from build123d import *

# Parameters (mm, degrees)
BOSS_EXTRUDE1_DEPTH = 15.86
SKETCH3_R           = 2.35
BOSS_EXTRUDE2_DEPTH = 1.8
SKETCH4_R           = 2.35
BOSS_EXTRUDE3_DEPTH = 1.8
SHELL1_T            = -1.4
SKETCH5_R           = 2.45
SKETCH5_R_2         = 1.45
BOSS_EXTRUDE4_DEPTH = 1.8
SKETCH6_R           = 3.05
SKETCH6_R_2         = 2.395
BOSS_EXTRUDE5_DEPTH = 1.55


with BuildPart() as part:
    # Sketch2 → Boss-Extrude1 (new body)
    with BuildSketch(Plane(origin=(0, 0, 0), x_dir=(0, 0, -1), z_dir=(1, 0, 0))):
        Polygon((0, 0), (0, 6.35), (-7.81, 6.35), (-7.81, 3.15), (-15.86, 3.15), (-15.86, 0), align=None)
    extrude(amount=BOSS_EXTRUDE1_DEPTH)

    # Sketch3 → Boss-Extrude2 (add)
    with BuildSketch(Plane(origin=(0, 6.35, 0), x_dir=(1, 0, 0), z_dir=(0, 1, 0))):
        with Locations(Location((3.98, -3.98, 0), (0, 0, 90))):
            Circle(SKETCH3_R)
        with Locations(Location((11.88, -3.98, 0), (0, 0, 90))):
            Circle(SKETCH3_R)
    extrude(amount=BOSS_EXTRUDE2_DEPTH)

    # Sketch4 → Boss-Extrude3 (add)
    with BuildSketch(Plane(origin=(0, 3.15, 0), x_dir=(1, 0, 0), z_dir=(0, 1, 0))):
        with Locations(Location((3.98, -11.88, 0), (0, 0, 90))):
            Circle(SKETCH4_R)
        with Locations(Location((11.88, -11.88, 0), (0, 0, 90))):
            Circle(SKETCH4_R)
    extrude(amount=BOSS_EXTRUDE3_DEPTH)

    # Shell1
    shell1_openings = [part.faces().sort_by_distance(p)[0] for p in [
        (7.93, 0, 7.93),
    ]]
    offset(amount=SHELL1_T, openings=shell1_openings, kind=Kind.INTERSECTION)

    # Sketch5 → Boss-Extrude4 (add)
    # profile 1 of 2: a face of its own
    with BuildSketch(Plane(origin=(0, 0, 0), x_dir=(-1, 0, 0), z_dir=(0, 0, -1))):
        with Locations(Location((-11.88, 3.9, 0), (0, 0, 90))):
            Circle(SKETCH5_R)
        with Locations((-11.88, 3.9)):
            Circle(SKETCH5_R_2, mode=Mode.SUBTRACT)
    # profile 2 of 2: a face of its own
    with BuildSketch(Plane(origin=(0, 0, 0), x_dir=(-1, 0, 0), z_dir=(0, 0, -1))):
        with Locations(Location((-3.92, 3.9, 0), (0, 0, 90))):
            Circle(SKETCH5_R)
        with Locations((-3.92, 3.9)):
            Circle(SKETCH5_R_2, mode=Mode.SUBTRACT)
    extrude(amount=BOSS_EXTRUDE4_DEPTH)

    # Sketch6 → Boss-Extrude5 (add)
    with BuildSketch(Plane.XZ.offset(-1.75)):
        with Locations(Location((7.93, 7.93, 0), (0, 0, 90))):
            Circle(SKETCH6_R)
        with Locations(Location((7.93, 7.93, 0), (0, 0, 90))):
            Circle(SKETCH6_R_2, mode=Mode.SUBTRACT)
    extrude(amount=BOSS_EXTRUDE5_DEPTH)


solid = part.part
Work out the finished part from the listing and answer in its coordinate system (mm). A direction names the side the tool comes from. Give positions to 0.01 mm unless a question says otherwise; leave off trailing zeros. Order: outer loops, then holes, each group sorted by start corner. A loop starts at its lowest first (then second) coordinate and runs counter-clockwise, first axis right, second up. Notation, with made-up numbers: (-31, 88.25) -> (-3, 88.25) arc R10 cw to (-3, 95.25) -> close; hole circle Ø7 at (77.5, 66). An arc over 180 degrees is marked (long way). Answer as a JSON object with one key per item and string values. Group by question number.
1. Section B-B on x = 7.93 is taken. Determine the outline of the cut face in (y, z) (3 decimals), plus the area to 3 significant figures.
2. Section A-A on y = 3.9 is taken. Determine the outline of the cut face in (x, z), plus the area to 3 significant figures.
3. The mould has two halves that part along Z. Classify faces 1 (the flat face through (8, 2, 0)), 2 (the cylindrical face through (7.01, 0.99, 10.84)), 3 (the flat face through (8, 4.95, 4)), 4 (the cylindrical face through (1.53, 3.37, -0.89)): released by +Z, released by -Z, zero draft, split by the parting line, or undercut.
4. Flat-ended cylindrical pins translate along their axes: pin 1 Ø1.9 at (x, y) = (9, 0.5) entering from -Z; pin 2 Ø1.5 at (x, z) = (5, 4) entering from -Y; pin 3 Ø3 at (x, z) = (10, 8) entering from -Y. Find the tip coordinate at first contact, or state that the pin passes through.
5. Section C-C on z = -0.5 is taken. Determine the outline of the cut face in (x, y), plus the area to 3 significant figures.
6. A tool of negligible diameter and unlimited length cuts with its end or side. For faces 5 (the flat face through (4, 3.55, 12)), 6 (the cylindrical face through (13.965, 4.037, 10.796)), 7 (the flat face through (4, 4, 0)), from which of +Z, -Z, +X, -X, +Y, -Y can it reach the whole face along a straight path? Write none if from no direction.
7. Section D-D on z = 3.98 is taken. Determine the outline of the cut face in (x, y).
8. Consider line 1 along X through (y, z) = (5.7, 3.98); line 2 along Z through (x, y) = (4.5, 3); line 3 along X through (y, z) = (1.25, 12.25). Determine where each line is inside the solid, lowest interval first. Write a range as [from, to].
Result sheet:
{
 "1": {"outline": "(0, 0) -> (6.35, 0) -> (6.35, 7.81) -> (3.15, 7.81) -> (3.15, 15.86) -> (0, 15.86) -> (0, 14.46) -> (1.75, 14.46) -> (1.75, 10.98) -> (0.2, 10.98) -> (0.2, 10.325) -> (1.75, 10.325) -> (1.75, 6.41) -> (4.95, 6.41) -> (4.95, 1.4) -> (0, 1.4) -> close; (0.2, 4.88) -> (1.75, 4.88) -> (1.75, 5.535) -> (0.2, 5.535) -> close", "area": "38.1 mm^2"},
 "2": {"outline": "(0, 0) -> (1.47, 0) -> (1.47, -1.8) -> (2.47, -1.8) -> (2.47, 0) -> (5.37, 0) -> (5.37, -1.8) -> (6.37, -1.8) -> (6.37, 0) -> (9.43, 0) -> (9.43, -1.8) -> (10.43, -1.8) -> (10.43, 0) -> (13.33, 0) -> (13.33, -1.8) -> (14.33, -1.8) -> (14.33, 0) -> (15.86, 0) -> (15.86, 7.81) -> (0, 7.81) -> close; circle Ø4.7 at (3.98, 11.88); circle Ø4.7 at (11.88, 11.88); hole (1.4, 1.4) -> (14.46, 1.4) -> (14.46, 6.41) -> (1.4, 6.41) -> close", "area": "100 mm^2"},
 "3": {"face 1": "released by -Z", "face 2": "undercut", "face 3": "undercut", "face 4": "zero draft"},
 "4": {"pin 1": "stops at z = 0", "pin 2": "stops at y = 4.95", "pin 3": "stops at y = 0.2"},
 "5": {"outline": "circle Ø4.9 at (3.92, 3.9); circle Ø4.9 at (11.88, 3.9); hole circle Ø2.9 at (3.92, 3.9); hole circle Ø2.9 at (11.88, 3.9)", "area": "24.5 mm^2"},
 "6": {"face 5": "-Y", "face 6": "+Y", "face 7": "-Z"},
 "7": {"outline": "(0, 0) -> (1.4, 0) -> (1.4, 4.95) -> (3.03, 4.95) -> (3.03, 6.75) -> (4.93, 6.75) -> (4.93, 4.95) -> (10.93, 4.95) -> (10.93, 6.75) -> (12.83, 6.75) -> (12.83, 4.95) -> (14.46, 4.95) -> (14.46, 0) -> (15.86, 0) -> (15.86, 6.35) -> (14.23, 6.35) -> (14.23, 8.15) -> (9.53, 8.15) -> (9.53, 6.35) -> (6.33, 6.35) -> (6.33, 8.15) -> (1.63, 8.15) -> (1.63, 6.35) -> (0, 6.35) -> close"},
 "8": {"line 1": "x = [0, 3.03], [4.93, 10.93], [12.83, 15.86]", "line 2": "z = [0, 1.4], [6.41, 11.08], [12.68, 15.86]", "line 3": "x = [0, 1.4], [14.46, 15.86]"}
}
